from build123d import *

# Parameters (mm, degrees)
F1_DEPTH = 10
F2_R     = 1.75
F3_DEPTH = 2
F4_R     = 1


with BuildPart() as f1:
    # F0 (on Front) → F1 (new body, symmetric)
    with BuildSketch(Plane.XZ):
        Polygon((-3, 3.5), (-1, 0), (1, 0), (3, 3.5), align=None)
    extrude(amount=F1_DEPTH, both=True)

    # F2 (on face) → F3 (cut)
    with BuildSketch(Plane.XY.offset(3.5)):
        Circle(F2_R)
    extrude(amount=-F3_DEPTH, mode=Mode.SUBTRACT)

    # F4
    f4_edges = [f1.edges().sort_by_distance(p)[0] for p in [
        (1, 0, 0),
        (-1, 0, 0),
    ]]
    fillet(f4_edges, radius=F4_R)


solid = f1.part
Design review of the part built by this model. Coordinates are the model's own, in mm. A direction names the side the tool comes from. Coordinates: 2 decimals unless noted, no trailing zeros. Loops run counter-clockwise (first coordinate to the right, second up) from the corner with the lowest first, then second, coordinate; pieces in that order, holes last. Notation, with made-up numbers: (-30, 33) -> (25, 33) arc R9 cw to (25, 41) -> close; hole circle Ø1 at (-14.5, 27). An arc over 180 degrees is marked (long way). Use a Markdown table: item, result. Add a question column.
Item 1: We need section A-A, the plane y = 0. Write out the cut boundary in (x, z), and give its area (3 significant figures).
Item 2: We need section C-C, the plane z = 3.3. Write out the cut boundary in (x, y).
Item 3: Wall thickness on L1, parallel to Y at x = 0, z = 2.95; L2, parallel to Z at x = 0.1, y = -0.25; L3, parallel to Y at x = -1.2, z = 3.1: over which ranges is each line inside the solid? List them lowest first. Write a range as from..to.
Item 4: The part is to be moulded in two halves that separate along X. For faces 3 (the flat face through (0, 0, 1.5)), 4 (the flat face through (-2.156, -0.14, 2.023)), 5 (the flat face through (-2, 0, 3.5)), say which applies: +X half, -X half, draft (parallel to the pull), parting line (faces both ways), or undercut.
Item 5: We need section D-D, the plane y = 3.75. Write out the cut boundary in (x, z).
Item 6: Clearance check with flat-ended pins moving along their axes: P1, Ø1.8, axis at x = -0.5, y = 0.5, coming from the +Z side; P2, Ø2, axis at y = 3.5, z = 3, coming from the -X side. State where each tip first meets the part, or that it passes through.
Item 7: Machinability: for faces 1 (the flat face through (2.13, -0.14, 1.98)), 2 (the cylindrical face through (1.617, -0.67, 2.514)), which of the approach directions +Z, -Z, +X, -X, +Y, -Y give a long, thin tool a straight path to every point of the face, cutting with its end or side? Answer none if there is none.
Item 8: We need section B-B, the plane x = 0. Write out the cut boundary in (y, z), and give its area (3 significant figures).
Numbers:
| question | item | result |
|---|---|---|
| 1 | outline | (-3, 3.5) -> (-1.29, 0.5) arc R1 ccw to (-0.42, 0) -> (0.42, 0) arc R1 ccw to (1.29, 0.5) -> (3, 3.5) -> (1.75, 3.5) -> (1.75, 1.5) -> (-1.75, 1.5) -> (-1.75, 3.5) -> close |
| 1 | area | 6.89 mm^2 |
| 2 | outline | (-2.89, -10) -> (2.89, -10) -> (2.89, 10) -> (-2.89, 10) -> close; hole circle Ø3.5 at (0, 0) |
| 3 | L1 | y = -10..-1.75, 1.75..10 |
| 3 | L2 | z = 0..1.5 |
| 3 | L3 | y = -10..-1.27, 1.27..10 |
| 4 | face 3 | undercut |
| 4 | face 4 | -X half |
| 4 | face 5 | draft |
| 5 | outline | (-3, 3.5) -> (-1.29, 0.5) arc R1 ccw to (-0.42, 0) -> (0.42, 0) arc R1 ccw to (1.29, 0.5) -> (3, 3.5) -> close |
| 6 | P1 | stops at z = 1.5 |
| 6 | P2 | stops at x = -3 |
| 7 | face 1 | -Z, +X, +Y, -Y |
| 7 | face 2 | +Z |
| 8 | outline | (-10, 0) -> (10, 0) -> (10, 3.5) -> (1.75, 3.5) -> (1.75, 1.5) -> (-1.75, 1.5) -> (-1.75, 3.5) -> (-10, 3.5) -> close |
| 8 | area | 63.0 mm^2 |
